Model file for the job. Use its own axes, mm. A direction names the side the tool comes from. Coordinates: 2 decimals unless noted, no trailing zeros. Write each loop counter-clockwise with the first axis right and the second up, starting at its lowest first coordinate (ties: lowest second). Pieces come first, ordered by that corner, then holes. Notation, with made-up numbers: (-10.75, 33) -> (-3.75, 33) arc R29 ccw to (-3.75, 70) -> close; hole circle Ø3 at (9, 89.25). An arc over 180 degrees is marked (long way). Answer as a JSON object with one key per item and string values. Group by question number.
from build123d import *

# Parameters (mm, degrees)
BOSS_EXTRUDE1_DEPTH = 16
SKETCH2_R           = 17
BOSS_EXTRUDE2_DEPTH = 17
SKETCH3_R           = 12.5
BOSS_EXTRUDE3_DEPTH = 24
SKETCH4_R           = 3
CUT_EXTRUDE1_DEPTH  = 97.093704268
BOSS_EXTRUDE5_DEPTH = 10
SKETCH7_R           = 82
CUT_EXTRUDE2_DEPTH  = 4
FILLET1_R           = 3


with BuildPart() as part:
    # Sketch1 → Boss-Extrude1 (new body)
    with BuildSketch(Plane(origin=(0, 0, 0), x_dir=(1, 0, 0), z_dir=(0, 1, 0))):
        with BuildLine():
            Line((0, 0), (23, 0))
            ThreePointArc((23, 0), (36.672989813, -16.671262796), (55.697765084, -6.525348371))
            Line((55.697765084, -6.525348371), (67, 0))
            Line((67, 0), (87, 0))
            Line((87, 0), (87, 7))
            Line((87, 7), (62, 7))
            ThreePointArc((62, 7), (45.688374241, 18.635635799), (26.997081597, 25.853165477))
            ThreePointArc((26.997081597, 25.853165477), (22.544359958, 24.799758331), (20.813284408, 20.564221286))
            Line((20.813284408, 20.564221286), (22, 7))
            Line((22, 7), (0, 7))
            Line((0, 7), (0, 0))
        make_face()
    extrude(amount=BOSS_EXTRUDE1_DEPTH)

    # Sketch2 → Boss-Extrude2 (add)
    with BuildSketch(Plane(origin=(0, 16, 0), x_dir=(1, 0, 0), z_dir=(0, 1, 0))):
        with Locations(Location((40, 0, 0), (0, 0, 116.765541629))):
            Circle(SKETCH2_R)
    extrude(amount=BOSS_EXTRUDE2_DEPTH)

    # Sketch3 → Boss-Extrude3 (add)
    with BuildSketch(Plane.XZ):
        with Locations(Location((40, 0, 0), (0, 0, 270))):
            Circle(SKETCH3_R)
    extrude(amount=BOSS_EXTRUDE3_DEPTH)

    # Sketch4 → Cut-Extrude1 (cut, through all)
    with BuildSketch(Plane(origin=(0, 0, -7), x_dir=(-1, 0, 0), z_dir=(0, 0, -1))):
        with Locations((-80.5, 8)):
            Circle(SKETCH4_R)
        with Locations((-6.5, 8)):
            Circle(SKETCH4_R)
    extrude(amount=-CUT_EXTRUDE1_DEPTH, mode=Mode.SUBTRACT)

    # Sketch5 → Boss-Extrude5 (add)
    with BuildSketch(Plane(origin=(0, 0, 0), x_dir=(1, 0, 0), z_dir=(0, 1, 0))):
        Polygon((67, 7), (73.302829045, 18.25023255), (82.899413644, 12.873843052), (86.320752416, 18.980760523), (68, 29.244776839), (55.512272379, 6.954811689), (55.512272379, 0), (67, 0), align=None)
    extrude(amount=-BOSS_EXTRUDE5_DEPTH)

    # Sketch7 → Cut-Extrude2 (cut)
    with BuildSketch(Plane(origin=(0, 13.5, 0), x_dir=(1, 0, 0), z_dir=(0, 1, 0))):
        with Locations((-0.4, -60)):
            Circle(SKETCH7_R)
    extrude(amount=CUT_EXTRUDE2_DEPTH, mode=Mode.SUBTRACT)

    # Fillet1
    fillet1_edges = [part.edges().sort_by_distance(p)[0] for p in [
        (47.655791005, 33, 15.178565943),
    ]]
    fillet(fillet1_edges, radius=FILLET1_R)


solid = part.part
(1) 3-axis set-ups, long thin cutter, end or side, ignore diameter. For faces 5 (the face through (78.03, -4.93, -15.6)), 6 (the face through (11, 7, 0)), 7 (the face through (61, -5, 0)): which of +Z, -Z, +X, -X, +Y, -Y reach the whole face in a straight line?
(2) Cut at B-B on y = 8. List the corners of the cut face in (x, z), plus the area to 3 significant figures.
(3) Wall check: probe 1 along Y at (x, z) = (29, 8.5); probe 2 along Y at (x, z) = (6.5, -4); probe 3 along X at (y, z) = (22, -11.5). Give the ranges that are in metal, low to high.
(4) Cut at D-D on x = 80.5. List the corners of the cut face in (y, z), plus the area to 3 significant figures.
(5) Cut at A-A on x = 6.5. List the corners of the cut face in (y, z), plus the area to 3 significant figures.
(6) Cut at C-C on y = -7.5. List the corners of the cut face in (x, z), plus the area to 3 significant figures.
(7) Pull direction Y, two halves, no side cores. Call faces 1 (the face through (40, 17.5, 1)), 2 (the face through (61.27, 7.89, 3.31)), 3 (the face through (3.64, 8.9, -3.55)), 4 (the face through (72, 0, -18)): released by +Y, released by -Y, zero draft, split by the parting line, or undercut.
(8) Pin check, flat tips, straight feed: pin 1 (4 mm diameter, centred on y = 5, z = 7, fed in from -X); pin 2 (18 mm diameter, centred on x = 78, z = -17.5, fed in from +Y); pin 3 (10 mm diameter, centred on x = 73, z = -6.5, fed in from +Y). Stop position of each tip, or through.
Results found:
{
 "1": {"face 5": "+Z, +Y, -Y", "face 6": "+Z, -X, +Y, -Y", "face 7": "+Z, +X, -Y"},
 "2": {"outline": "(0, -7) -> (3.5, -7) -> (3.5, 0) -> (0, 0) -> close; (9.5, -7) -> (22, -7) -> (20.81, -20.56) arc R5 ccw to (27, -25.85) arc R80 ccw to (62, -7) -> (77.5, -7) -> (77.5, 0) -> (67, 0) -> (55.7, 6.53) arc R17 ccw to (23, 0) -> (9.5, 0) -> close; (83.5, -7) -> (87, -7) -> (87, 0) -> (83.5, 0) -> close", "area": "1,510 mm²"},
 "3": {"probe 1": "y = 0 to 13.5, 17.5 to 33", "probe 2": "y = 0 to 5, 11 to 13.5", "probe 3": "x = 27.48 to 52.52"},
 "4": {"outline": "(-10, -22.24) -> (0, -22.24) -> (0, -14.22) -> (-10, -14.22) -> close; (0, -7) -> (5, -7) -> (5, 0) -> (0, 0) -> close; (11, -7) -> (16, -7) -> (16, 0) -> (11, 0) -> close", "area": "150 mm²"},
 "5": {"outline": "(0, -7) -> (5, -7) -> (5, 0) -> (0, 0) -> close; (11, -7) -> (13.5, -7) -> (13.5, 0) -> (11, 0) -> close", "area": "52.5 mm²"},
 "6": {"outline": "circle Ø25 at (40, 0); (55.51, -6.95) -> (68, -29.24) -> (86.32, -18.98) -> (82.9, -12.87) -> (73.3, -18.25) -> (67, -7) -> (67, 0) -> (55.51, 0) -> close", "area": "875 mm²"},
 "7": {"face 1": "undercut", "face 2": "zero draft", "face 3": "undercut", "face 4": "released by +Y"},
 "8": {"pin 1": "stops at x = 23.75", "pin 2": "stops at y = 0", "pin 3": "stops at y = 16"}
}
